Source: three-view drawing plus pictorial views. Frame: mm from the lowest corner of the part. A direction names the side the tool comes from. Coordinates: 2 decimals unless noted, no trailing zeros. Write each loop counter-clockwise with the first axis right and the second up, starting at its lowest first coordinate (ties: lowest second). Pieces come first, ordered by that corner, then holes. Notation, with made-up numbers: (2.25, 81.5) -> (37.25, 81.5) arc R18 cw to (37.25, 90.5) -> close; hole circle Ø2 at (30, 37). An arc over 180 degrees is marked (long way). One line per item, written item: value.
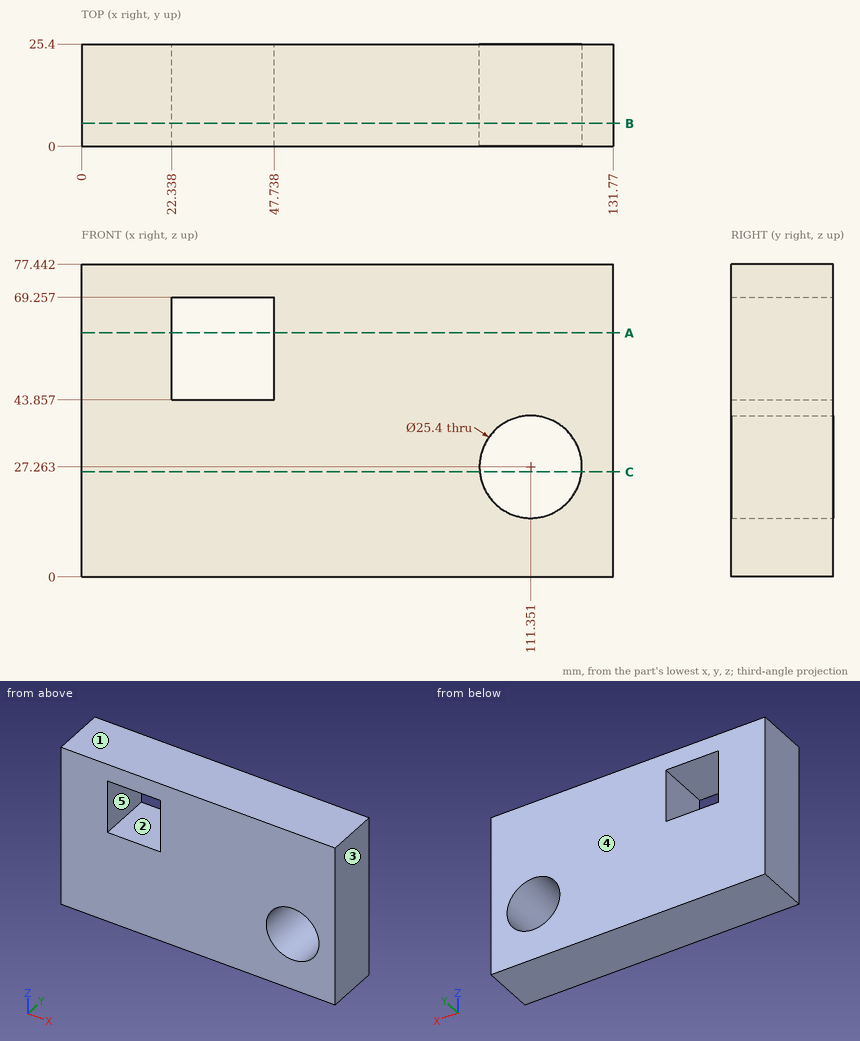
(1) Line query: line 1 (Z direction, x = 33, y = 3.75); line 2 (X direction, y = 15, z = 28); line 3 (X direction, y = 11.5, z = 50). Output: solid intervals per line, ascending. Write a range as [from, to].
Responses:
line 1: z = [0, 43.86], [69.26, 77.44]
line 2: x = [0, 98.67], [124.03, 131.77]
line 3: x = [0, 22.34], [47.74, 131.77]
(2) Reachability of the marked faces 1 and 2 from +Z, -Z, +X, -X, +Y, -Y: full face, straight path, thin tool, end or side. Return the list, or none.
Responses:
face 1: +Z, +X, -X, +Y, -Y
face 2: +Y, -Y
(3) Section C-C (z = 26). Return the cut outline in (x, y), then the cut area to 4 significant figures.
Responses:
outline: (0, 0) -> (98.71, 0) -> (98.71, 25.4) -> (0, 25.4) -> close; (123.99, 0) -> (131.77, 0) -> (131.77, 25.4) -> (123.99, 25.4) -> close
area: 2,705 mm2
(4) Section B-B (y = 5.75). Return the cut outline in (x, z).
Responses:
outline: (0, 0) -> (131.77, 0) -> (131.77, 77.44) -> (0, 77.44) -> close; hole (22.34, 43.86) -> (47.74, 43.86) -> (47.74, 69.26) -> (22.34, 69.26) -> close; hole circle Ø25.4 at (111.35, 27.26)
(5) Pull-direction query (X, two-part tool) for the marked faces 3, 4 and 5; classes: released by +X, released by -X, zero draft, split by the parting line, or undercut.
Responses:
face 3: released by +X
face 4: zero draft
face 5: undercut
(6) Section A-A (z = 60.5). Return the cut outline in (x, y).
Responses:
outline: (0, 0) -> (22.34, 0) -> (22.34, 25.4) -> (0, 25.4) -> close; (47.74, 0) -> (131.77, 0) -> (131.77, 25.4) -> (47.74, 25.4) -> close
